```python
from build123d import *

# Parameters (mm, degrees)
REFERENCE_HEAD_START           = -1
SKETCH1_R                      = 2
REFERENCE_HEAD_DEPTH           = 1
SKETCH2_R                      = 1
REFERENCE_SHANK_DEPTH          = 7.5
SKETCH3_R                      = 1.01
SKETCH3_R_2                    = 0.8
M1P6_END_THREAD_ENVELOPE_DEPTH = 2.3


with BuildPart() as part:
    # Sketch1 → Reference_Head (new body)
    with BuildSketch(Plane.XY.offset(REFERENCE_HEAD_START)):
        Circle(SKETCH1_R)
    extrude(amount=REFERENCE_HEAD_DEPTH)

    # Sketch2 → Reference_Shank (add)
    with BuildSketch(Plane.XY):
        Circle(SKETCH2_R)
    extrude(amount=REFERENCE_SHANK_DEPTH)

    # Sketch3 → M1p6_End_Thread_Envelope (cut)
    with BuildSketch(Plane.XY.offset(7.5)):
        Circle(SKETCH3_R)
        Circle(SKETCH3_R_2, mode=Mode.SUBTRACT)
    extrude(amount=-M1P6_END_THREAD_ENVELOPE_DEPTH, mode=Mode.SUBTRACT)


solid = part.part
```
Geometry check sheet. Reference: the model listing, model coordinates, mm. A direction names the side the tool comes from. Give positions to 0.01 mm unless a question says otherwise; leave off trailing zeros. Order: outer loops, then holes, each group sorted by start corner. A loop starts at its lowest first (then second) coordinate and runs counter-clockwise, first axis right, second up.
1. Section check A-A, the plane x = 0. Enter the section's corners in (y, z), and give its area (3 significant figures).
2. Gauge pin test, flat end, axial feed: pin 1 Ø1.5 at (y, z) = (0.5, 3) entering from -X. Record the tip position at first contact, or that the pin passes through.
3. Section check C-C, the plane z = 2.75. Enter the section's corners in (x, y).
4. Section check D-D, the plane z = 5.5. Enter the section's corners in (x, y), and give its area (3 significant figures).
5. Access from +Z, -Z, +X, -X, +Y, -Y to the whole of each face (thin tool, end or side, straight path). Record for faces 1 (the face through (-0.434, -1.952, -0.507)), 2 (the face through (-0.63, -0.49, 6.37)).
6. Thickness scan on L1, parallel to Z at x = 0.6, y = 1.5; L2, parallel to Y at x = -0.45, z = 0.25; L3, parallel to X at y = -0.75, z = 3.75. Record the ranges inside material, lowest first.
Values follow:
1. outline: (-2, -1) - (2, -1) - (2, 0) - (1, 0) - (1, 5.2) - (0.8, 5.2) - (0.8, 7.5) - (-0.8, 7.5) - (-0.8, 5.2) - (-1, 5.2) - (-1, 0) - (-2, 0) - close
1. area: 18.1 mm2
2. pin 1: stops at x = -1
3. outline: circle Ø2 at (0, 0)
4. outline: circle Ø1.6 at (0, 0)
4. area: 2.01 mm2
5. face 1: +Z, -Z
5. face 2: +Z
6. L1: z = -1 to 0
6. L2: y = -0.89 to 0.89
6. L3: x = -0.66 to 0.66
